Input: part model. Units: mm. Frame: model coordinates. Face numbers are marked on the shaded views. A direction names the side the tool comes from. Coordinates: 2 decimals unless noted, no trailing zeros. Order: outer loops, then holes, each group sorted by start corner. A loop starts at its lowest first (then second) coordinate and runs counter-clockwise, first axis right, second up.
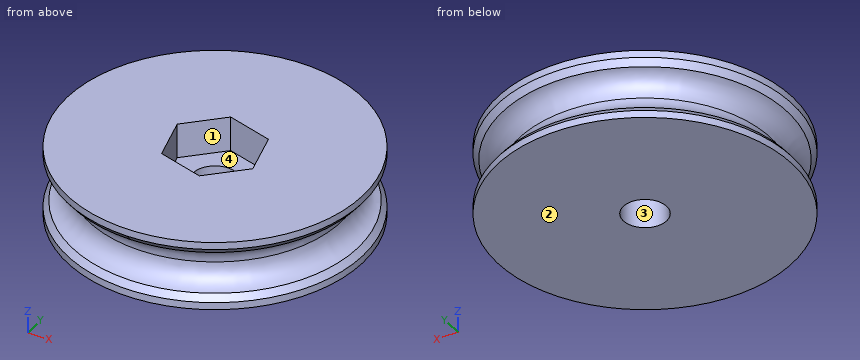
from build123d import *

# Parameters (mm, degrees)
F0_R        = 17
F1_DEPTH    = 4
F2_R        = 2.5
F3_DEPTH    = 25
F5_DEPTH    = 4
F6_R        = 2.5
F8_T2_ANGLE = 270
F8_T4_ANGLE = 90
F8_T6_ANGLE = 90
F8_T8_ANGLE = 270


# Not quite as in the source:
# - a fillet or chamfer that OpenCascade refuses, or shapes differently, is made with other operations: its cross-section is extruded or revolved along the edge and cut away or added


with BuildPart() as f1:
    # F0 (on Top) → F1 (new body, symmetric)
    with BuildSketch(Plane.XY):
        Circle(F0_R)
    extrude(amount=F1_DEPTH, both=True)

    # F2 (on face) → F3 (cut)
    with BuildSketch(Plane.XY.offset(4)):
        Circle(F2_R)
    extrude(amount=-F3_DEPTH, mode=Mode.SUBTRACT)

    # F4 (on face) → F5 (cut)
    with BuildSketch(Plane.XY.offset(4)):
        Polygon((5.2209928438, -1.4814071211), (3.8934326221, 3.7808088751), (-1.3275602216, 5.2622159963), (-5.2209928438, 1.4814071211), (-3.8934326221, -3.7808088751), (1.3275602216, -5.2622159963), align=None)
    extrude(amount=-F5_DEPTH, mode=Mode.SUBTRACT)

    # F6 (on Right) → F7 (revolve, cut)
    with BuildSketch(Plane.YZ):
        with Locations((-17, 0)):
            Circle(F6_R)
    revolve(axis=Axis((0, 0, 0), (0, 0, 1)), mode=Mode.SUBTRACT)

    # F8: chamfer of 0.75 on 4 edges, made by hand

    # F8_s1 → F8_t2 (revolve, cut)
    with BuildSketch(Plane.YZ):
        with BuildLine():
            Line((-17, -3.1622776602), (-16.4230769231, -2.4325212771))
            ThreePointArc((-16.4230769231, -2.4325212771), (-16.6989227011, -2.4818042751), (-17, -2.5))
            Line((-17, -2.5), (-17, -3.1622776602))
        make_face()
    revolve(axis=Axis((0, 0, -2.5), (0, 0, -1)), revolution_arc=F8_T2_ANGLE, mode=Mode.SUBTRACT)

    # F8_s3 → F8_t4 (revolve, cut)
    with BuildSketch(Plane.XZ):
        with BuildLine():
            Line((17, -3.1622776602), (16.4230769231, -2.4325212771))
            ThreePointArc((16.4230769231, -2.4325212771), (16.6989227011, -2.4818042751), (17, -2.5))
            Line((17, -2.5), (17, -3.1622776602))
        make_face()
    revolve(axis=Axis((0, 0, -2.5), (0, 0, -1)), revolution_arc=F8_T4_ANGLE, mode=Mode.SUBTRACT)

    # F8_s5 → F8_t6 (revolve, cut)
    with BuildSketch(Plane.XZ):
        with BuildLine():
            Line((16.4230769231, 2.4325212771), (17, 3.1622776602))
            Line((17, 3.1622776602), (17, 2.5))
            ThreePointArc((17, 2.5), (16.6989227011, 2.4818042751), (16.4230769231, 2.4325212771))
        make_face()
    revolve(axis=Axis((0, 0, 2.5), (0, 0, -1)), revolution_arc=F8_T6_ANGLE, mode=Mode.SUBTRACT)

    # F8_s7 → F8_t8 (revolve, cut)
    with BuildSketch(Plane.YZ):
        with BuildLine():
            Line((-16.4230769231, 2.4325212771), (-17, 3.1622776602))
            Line((-17, 3.1622776602), (-17, 2.5))
            ThreePointArc((-17, 2.5), (-16.6989227011, 2.4818042751), (-16.4230769231, 2.4325212771))
        make_face()
    revolve(axis=Axis((0, 0, 2.5), (0, 0, -1)), revolution_arc=F8_T8_ANGLE, mode=Mode.SUBTRACT)


solid = f1.part
Item 1: Draft query along X for the marked faces 1 and 2. Return one class per face: pulls with the +X half, pulls with the -X half, needs draft (parallel to the pull), parting line crosses it, or undercut.
Response values:
face 1: undercut
face 2: needs draft
Item 2: Ray query, probe 1 along Z at (x, y) = (-13.5, -6.5); probe 2 along X at (y, z) = (1.5, -0.75); probe 3 along Z at (x, y) = (4, -2.5). Return the intervals inside material, ascending.
Response values:
probe 1: z = -4 to -1.48, 1.48 to 4
probe 2: x = -14.54 to -2, 2 to 14.54
probe 3: z = -4 to 0
Item 3: Access query for the marked faces 3 and 4. Directions: +Z, -Z, +X, -X, +Y, -Y. A direction counts if a zero-diameter tool reaches every point of the face in a straight line with its end or side. Return the directions, or none.
Response values:
face 3: +Z, -Z
face 4: +Z
Item 4: Pin query (flat end, axial travel): pin 1 Ø1 at (x, z) = (-4, 2) entering from -Y; pin 2 Ø6 at (x, y) = (0, 0) entering from +Z; pin 3 Ø8.5 at (x, y) = (0.5, 0.5) entering from +Z. Return the tip coordinate at first contact, or that it passes through.
Response values:
pin 1: stops at y = -16
pin 2: stops at z = 0
pin 3: stops at z = 4
Item 5: Cut plane A-A on z = -2. Return loops of the section in (x, y).
Response values:
outline: circle Ø31 at (0, 0); hole circle Ø5 at (0, 0)
